Check sheet for the modelled part. Datum: model origin and axes. Units: mm. Round coordinates to 2 decimals unless told otherwise and drop trailing zeros. Loops run counter-clockwise (first coordinate to the right, second up) from the corner with the lowest first, then second, coordinate; pieces in that order, holes last. Notation, with made-up numbers: (72, 39.5) -> (98, 39.5) arc R8 ccw to (98, 45.5) -> close; hole circle Ø3 at (12, 40.5). An arc over 180 degrees is marked (long way). One line per item, written item: value. Start each with the question number.
1. Material ranges on L1, parallel to Z at x = 0.85, y = -27.5; L2, parallel to Y at x = 1.45, z = 47; L3, parallel to Z at x = 1.2, y = 137.3, recorded low to high.
2. Cross-section at B-B on z = -4.5. Record the cut outline in (x, y), then the cut area to 3 significant figures.
3. Cross-section at C-C on x = 1.15. Count the separate pieces of the cut face and the enclosed holes in it, then the cut area to 3 significant figures.
4. Go/stop test with a flat-tipped pin: pin 1 (2.5 mm diameter, centred on y = -107.5, z = -60, fed in from -X). Record where the tip stops, or that it passes through.
5. Cross-section at A-A on y = 35. Record the cut outline in (x, z).
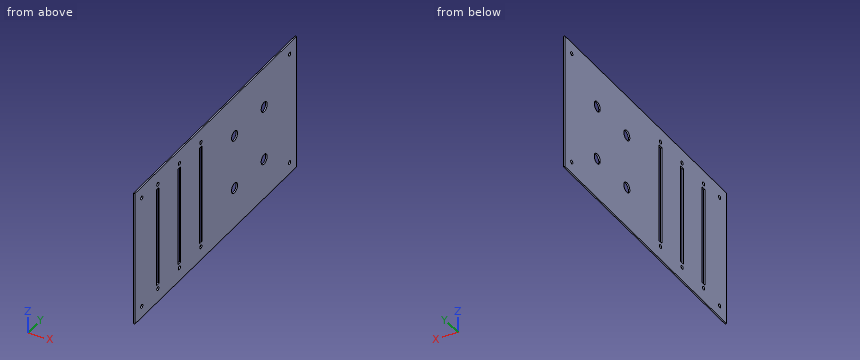
from build123d import *

# Parameters (mm, degrees)
SKETCH1_W                            = 300
SKETCH1_H                            = 150
BOSS_EXTRUDE1_DEPTH                  = 1.52
F_4_0_4_DIAMETER_HOLE1_D             = 4
MIRROR2_AT_THE_SECOND_PLANE_COPY_1_D = 4
SKETCH14_W                           = 5
SKETCH14_H                           = 110
CUT_EXTRUDE2_DEPTH                   = 168.711986453
F_4_0_4_DIAMETER_HOLE2_D             = 4
SKETCH22_W                           = 5
SKETCH22_H                           = 110
CUT_EXTRUDE3_DEPTH                   = 168.711986453
SKETCH23_W                           = 5
SKETCH23_H                           = 110
CUT_EXTRUDE4_DEPTH                   = 168.711986453
F_4_0_4_DIAMETER_HOLE3_D             = 4
F_4_0_4_DIAMETER_HOLE4_D             = 4
F_11_0_11_DIAMETER_HOLE1_D           = 11


with BuildPart() as part:
    # Sketch1 → Boss-Extrude1 (new body)
    with BuildSketch(Plane.YZ):
        Rectangle(SKETCH1_W, SKETCH1_H)
    extrude(amount=BOSS_EXTRUDE1_DEPTH)

    # Ø4.0 (4) Diameter Hole1 (through all)
    with Locations(Plane.YZ.offset(1.52)):
        with Locations((-137.3, 62.3)):
            f_4_0_4_diameter_hole1 = Hole(F_4_0_4_DIAMETER_HOLE1_D / 2)

    # Mirror2: Ø4.0 (4) Diameter Hole1 across plane
    add(f_4_0_4_diameter_hole1.mirror(Plane.ZX), mode=Mode.SUBTRACT)

    # Mirror2 at the second plane: Ø4.0 (4) Diameter Hole1 across plane
    add(f_4_0_4_diameter_hole1.mirror(Plane.XY), mode=Mode.SUBTRACT)

    # Mirror2 at the second plane copy 1 (through all)
    with Locations(Plane(origin=(1.52, 0, 0), x_dir=(0, -1, 0), z_dir=(1, 0, 0))):
        with Locations((-137.3, 62.3)):
            Hole(MIRROR2_AT_THE_SECOND_PLANE_COPY_1_D / 2)

    # Sketch14 → Cut-Extrude2 (cut, through all)
    with BuildSketch(Plane.YZ.offset(1.52)):
        with Locations((-107.5, 0)):
            Rectangle(SKETCH14_W, SKETCH14_H)
    extrude(amount=-CUT_EXTRUDE2_DEPTH, mode=Mode.SUBTRACT)

    # Ø4.0 (4) Diameter Hole2 (through all)
    with Locations(Plane.YZ.offset(1.52)):
        with Locations((-107.5, 60)):
            f_4_0_4_diameter_hole2 = Hole(F_4_0_4_DIAMETER_HOLE2_D / 2)

    # Mirror4: Ø4.0 (4) Diameter Hole2 across plane
    add(f_4_0_4_diameter_hole2.mirror(Plane.XY), mode=Mode.SUBTRACT)

    # Sketch22 → Cut-Extrude3 (cut, through all)
    with BuildSketch(Plane.YZ.offset(1.52)):
        with Locations((-67.5, 0)):
            Rectangle(SKETCH22_W, SKETCH22_H)
    extrude(amount=-CUT_EXTRUDE3_DEPTH, mode=Mode.SUBTRACT)

    # Sketch23 → Cut-Extrude4 (cut, through all)
    with BuildSketch(Plane.YZ.offset(1.52)):
        with Locations((-27.5, 0)):
            Rectangle(SKETCH23_W, SKETCH23_H)
    extrude(amount=-CUT_EXTRUDE4_DEPTH, mode=Mode.SUBTRACT)

    # Ø4.0 (4) Diameter Hole3 (through all)
    with Locations(Plane.YZ.offset(1.52)):
        with Locations((-67.5, 60)):
            f_4_0_4_diameter_hole3 = Hole(F_4_0_4_DIAMETER_HOLE3_D / 2)

    # Mirror5: Ø4.0 (4) Diameter Hole3 across plane
    add(f_4_0_4_diameter_hole3.mirror(Plane.XY), mode=Mode.SUBTRACT)

    # Ø4.0 (4) Diameter Hole4 (through all)
    with Locations(Plane.YZ.offset(1.52)):
        with Locations((-27.5, 60)):
            f_4_0_4_diameter_hole4 = Hole(F_4_0_4_DIAMETER_HOLE4_D / 2)

    # Mirror6: Ø4.0 (4) Diameter Hole4 across plane
    add(f_4_0_4_diameter_hole4.mirror(Plane.XY), mode=Mode.SUBTRACT)

    # Ø11.0 (11) Diameter Hole1 (through all)
    with Locations(Plane.YZ.offset(1.52)):
        with Locations((35, 30), (90, 30)):
            f_11_0_11_diameter_hole1 = Hole(F_11_0_11_DIAMETER_HOLE1_D / 2)

    # Mirror7: Ø11.0 (11) Diameter Hole1 across plane
    add(f_11_0_11_diameter_hole1.mirror(Plane.XY), mode=Mode.SUBTRACT)


solid = part.part
Taken from the geometry:
1. L1: z = -75 to -62, -58 to -55, 55 to 58, 62 to 75
1. L2: y = -150 to -110, -105 to -70, -65 to -30, -25 to 150
1. L3: z = -75 to -64.3, -60.3 to 60.3, 64.3 to 75
2. outline: (0, -150) -> (1.52, -150) -> (1.52, -110) -> (0, -110) -> close; (0, -105) -> (1.52, -105) -> (1.52, -70) -> (0, -70) -> close; (0, -65) -> (1.52, -65) -> (1.52, -30) -> (0, -30) -> close; (0, -25) -> (1.52, -25) -> (1.52, 150) -> (0, 150) -> close
2. area: 433 mm2
3. separate pieces: 1
3. enclosed holes: 17
3. area: 42,800 mm2
4. pin 1: passes through
5. outline: (0, -75) -> (1.52, -75) -> (1.52, -35.5) -> (0, -35.5) -> close; (0, -24.5) -> (1.52, -24.5) -> (1.52, 24.5) -> (0, 24.5) -> close; (0, 35.5) -> (1.52, 35.5) -> (1.52, 75) -> (0, 75) -> close
